The figure shows three views and two pictorial views of one solid part (mm, origin at its lowest corner). Answer the questions. Round coordinates to 2 decimals unless told otherwise and drop trailing zeros. Order: outer loops, then holes, each group sorted by start corner. A loop starts at its lowest first (then second) coordinate and runs counter-clockwise, first axis right, second up. Notation, with made-up numbers: (56.5, 2) -> (112.5, 2) arc R7 cw to (112.5, 11) -> close; hole circle Ø11 at (3, 10). An arc over 180 degrees is marked (long way). Answer as a JSON object with one key per item and string values. Group by question number.
Item 1: Consider probe 1 along X at (y, z) = (22.5, 6.5); probe 2 along Y at (x, z) = (79, 7); probe 3 along Z at (x, y) = (78.5, 16.5). Determine where each line is inside the solid, lowest interval first. Write a range as from..to.
Item 2: Section D-D, the plane y = 22 is taken. Write down the section's boundary in (x, z), plus the area to 3 significant figures.
Item 3: Given P1, Ø1.8, axis at y = 32, z = 9.5, coming from the -X side; P2, Ø4, axis at x = 124.5, y = 89.5, coming from the -Z side; P3, Ø5, axis at y = 58, z = 9, coming from the +X side; P4, Ø1.5, axis at x = 25, y = 100.5, coming from the +Z side, each flat-ended and moving along its own axis, determine where each tip first touches the part or whether it passes through.
Item 4: Section B-B, the plane y = 91 is taken. Write down the section's boundary in (x, z), plus the area to 3 significant figures.
Item 5: Section C-C, the plane x = 64 is taken. Write down the section's boundary in (y, z), plus the area to 3 significant figures.
Item 6: Section A-A, the plane z = 9.75 is taken. Write down the section's boundary in (x, y).
Item 7: The mould has two halves that part along X. Classify the marked faces 1, 2 and 3: pulls with the +X half, pulls with the -X half, needs draft (parallel to the pull), parting line crosses it, or undercut.
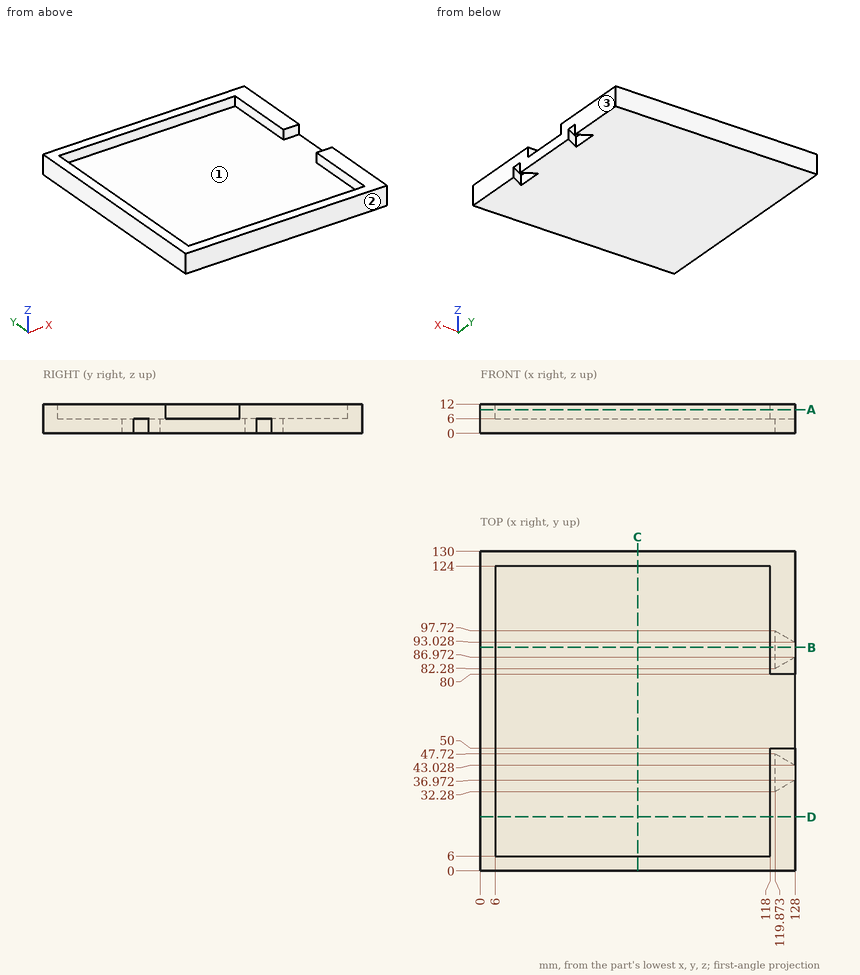
Values found:
{
 "1": {"probe 1": "0..6, 118..128", "probe 2": "0..6, 124..130", "probe 3": "0..6"},
 "2": {"outline": "(0, 0) -> (128, 0) -> (128, 12) -> (118, 12) -> (118, 6) -> (6, 6) -> (6, 12) -> (0, 12) -> close", "area": "864 mm2"},
 "3": {"P1": "x = 0", "P2": "z = 6", "P3": "x = 6", "P4": "z = 6"},
 "4": {"outline": "(0, 0) -> (119.87, 0) -> (119.87, 6) -> (128, 6) -> (128, 12) -> (118, 12) -> (118, 6) -> (6, 6) -> (6, 12) -> (0, 12) -> close", "area": "815 mm2"},
 "5": {"outline": "(0, 0) -> (130, 0) -> (130, 12) -> (124, 12) -> (124, 6) -> (6, 6) -> (6, 12) -> (0, 12) -> close", "area": "852 mm2"},
 "6": {"outline": "(0, 0) -> (128, 0) -> (128, 50) -> (118, 50) -> (118, 6) -> (6, 6) -> (6, 124) -> (118, 124) -> (118, 80) -> (128, 80) -> (128, 130) -> (0, 130) -> close"},
 "7": {"face 1": "undercut", "face 2": "needs draft", "face 3": "pulls with the +X half"}
}
